Part model, mm, in its own coordinate system. Face numbers are marked on the shaded views. A direction names the side the tool comes from. Round coordinates to 2 decimals unless told otherwise and drop trailing zeros. Write each loop counter-clockwise with the first axis right and the second up, starting at its lowest first coordinate (ties: lowest second). Pieces come first, ordered by that corner, then holes. Notation, with made-up numbers: M 88.25,33.25 L 122.25,33.25 A29 cw 122.25,61.25 Z; hole C 0.25,80 d7. An arc over 180 degrees is marked long. Answer as a JSON object with one key per item and string values. Group by question number.
1. Band-saw the part on D-D, the plane y = -0.25. Write the cut outline in (x, z), plus the area to 3 significant figures.
2. Drill centre lines: line 1 (Z direction, x = 0, y = 7.3); line 2 (X direction, y = 8, z = 0.5). Where is each one in solid material? Low to high. Write a range as from..to.
3. Band-saw the part on C-C, the plane y = 7.75. Write the cut outline in (x, z), plus the area to 3 significant figures.
4. Band-saw the part on B-B, the plane x = 0. Write the cut outline in (y, z).
5. Two-plate mould, pull along Z, no slides. Class the marked faces 1, 2 and 3: +Z half, -Z half, draft (parallel to the pull), parting line (faces both ways), or undercut.
6. Drop flat-ended pins along their axis: pin 1 (0.5 mm diameter, centred on y = 9, z = 2, fed in from -X); pin 2 (1.9 mm diameter, centred on x = 0.5, z = 0, fed in from +Y); pin 3 (0.5 mm diameter, centred on y = 8.5, z = -2, fed in from +X). Give the stop position or say it passes through.
7. Which spindle directions (+Z, -Z, +X, -X, +Y, -Y) get a long thin tool onto all of the face, cutting with end or side? Do the marked faces 4, 5 and 6. Say none if no direction does.
8. Band-saw the part on A-A, the plane z = 0. Write the cut outline in (x, y).
Autodesk Inventor part; units mm, degrees
ref_plane "YZ Plane" through (0, 0, 0) normal (1, 0, 0) x (0, 1, 0)
ref_plane "XZ Plane" through (0, 0, 0) normal (0, 1, 0) x (-1, 0, 0)
ref_plane "XY Plane" through (0, 0, 0) normal (0, 0, 1) x (1, 0, 0)
sketch "スケッチ1" plane through (0, 0, 0) normal (0, 0, 1) x (1, 0, 0)
  line L0 (0, -4.25) -> (0.9, -4.25)
  line L1 (0.9, -4.25) -> (1.2, -3.95)
  line L2 (1.2, -3.95) -> (1.2, 1.25)
  line L3 (1.2, 1.25) -> (1.5, 1.25)
  line L4 (1.5, 1.25) -> (1.5, 1.75)
  line L5 (1.5, 1.75) -> (2.7, 1.75)
  line L6 (3, 8.95) -> (2.7, 9.25)
  line L7 (2.7, 9.25) -> (1.5, 9.25)
  line L8 (1.5, 9.25) -> (1.2, 8.95)
  line L9 (0, 7.4044) -> (0, -7.4044) construction
  line L10 (0, -4.25) -> (0, 4.25)
  line L11 (0, 4.25) -> (1.2, 4.25)
  line L12 (1.2, 4.25) -> (1.2, 8.95)
  line L13 (2.7, 1.75) -> (3, 2.05)
  line L14 (3, 2.05) -> (3, 8.95)
  point P0 (0, 0)
  point P1 (0, 0)
  point P2 (0, 0)
  dimension "d0" = 2.4
  dimension "d1" = 6
  dimension "d2" = 0.3
  dimension "d3" = 0.3
  dimension "d4" = 3
  dimension "d5" = 0.5
  dimension "d6" = 7.5
  dimension "d7" = 0.3
  dimension "d8" = 2.4
  dimension "d9" = 5
  dimension "d10" = 0.3
  dimension "d11" = 0.3
  dimension "d12" = 0.3
  dimension "d13" = 0.3
  dimension "d14" = 6
revolve "回転1" add sketch "スケッチ1" angle 360 about axis through (0, 7.4044, 0) along (0, -1, 0)
sketch "スケッチ2" plane through (0, 9.25, 0) normal (0, 1, 0) x (1, 0, 0)
  line L0 (-0.5, 3) -> (0.5, 3)
  line L1 (0.5, 3) -> (0.5, -3)
  line L2 (0.5, -3) -> (-0.5, -3)
  line L3 (-0.5, -3) -> (-0.5, 3)
  line L4 (-0.5, 3) -> (0.5, -3) construction
  line L5 (0.5, 3) -> (-0.5, -3) construction
  circle A0 centre (0, 0) radius 3
  point P0 (0, 0)
  point P1 (0.5, 2.958)
  point P2 (-0.5, 2.958)
  point P3 (-0.5, -2.958)
  point P4 (0.5, -2.958)
  dimension "d16" = 1
extrude "押し出し1" cut sketch "スケッチ2" against normal blind 1 contours A0 L1 L3
equation "\"d3\" = d2"
equation "\"d10\" = d7"
equation "\"d11\" = d7"
equation "\"d12\" = d11"
equation "\"d13\" = d12"
properties part number "BRU-307_5S" material "ステンレス鋼 AISI 304"
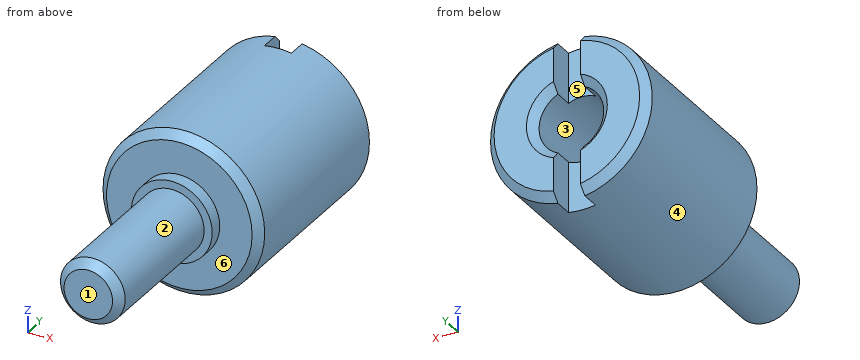
Worked answers:
{
 "1": {"outline": "C 0,0 d2.4", "area": "4.52 mm^2"},
 "2": {"line 1": "z = -3..-1.2, 1.2..3", "line 2": "x = -2.96..-1.09, 1.09..2.96"},
 "3": {"outline": "C 0,0 d6; hole C 0,0 d2.4", "area": "23.8 mm^2"},
 "4": {"outline": "M -4.25,-0.9 L -3.95,-1.2 L 1.25,-1.2 L 1.25,-1.5 L 1.75,-1.5 L 1.75,-2.7 L 2.05,-3 L 8.25,-3 L 8.25,-1.2 L 4.25,-1.2 L 4.25,1.2 L 8.25,1.2 L 8.25,3 L 2.05,3 L 1.75,2.7 L 1.75,1.5 L 1.25,1.5 L 1.25,1.2 L -3.95,1.2 L -4.25,0.9 Z"},
 "5": {"face 1": "draft", "face 2": "parting line", "face 3": "undercut"},
 "6": {"pin 1": "stops at x = -2.43", "pin 2": "stops at y = 9.2", "pin 3": "stops at x = 2.44"},
 "7": {"face 4": "+Y, -Y", "face 5": "+Z, -Z, +Y", "face 6": "-Y"},
 "8": {"outline": "M -3,2.05 L -2.7,1.75 L -1.5,1.75 L -1.5,1.25 L -1.2,1.25 L -1.2,-3.95 L -0.9,-4.25 L 0.9,-4.25 L 1.2,-3.95 L 1.2,1.25 L 1.5,1.25 L 1.5,1.75 L 2.7,1.75 L 3,2.05 L 3,8.95 L 2.7,9.25 L 1.5,9.25 L 1.2,8.95 L 1.2,4.25 L -1.2,4.25 L -1.2,8.95 L -1.5,9.25 L -2.7,9.25 L -3,8.95 Z"}
}
